Here's how the part is built. I have some questions about the finished solid (model axes, mm). Face numbers are marked on the shaded views. A direction names the side the tool comes from. Round coordinates to 2 decimals unless told otherwise and drop trailing zeros. Order: outer loops, then holes, each group sorted by start corner. A loop starts at its lowest first (then second) coordinate and runs counter-clockwise, first axis right, second up. Notation, with made-up numbers: M 37.25,54 L 64.25,54 A27 cw 64.25,90 Z; hole C 54.25,25 d9. An arc over 180 degrees is marked long. Write item = value, one per line. Start each with the question number.
Item 1: I'm going to push a flat-ended pin straight in: P1, Ø1, axis at y = 1.5, z = 0, coming from the -X side. Where does the tip first touch, or does it pass through?
Item 2: I want a section at C-C, the plane y = 1.95. State how many separate pieces and enclosed holes the cut face has, plus the area to 3 significant figures.
Item 3: We'd pull the mould along Z, two halves only. Please class the marked faces 4, 5 and 6: pulls with the +Z half, pulls with the -Z half, needs draft (parallel to the pull), parting line crosses it, or undercut.
Item 4: I want a section at B-B, the plane z = 0. List the corners of the cut face in (x, y) for me (1 decimal).
Item 5: For the marked faces 1, 2 and 3, which set-ups out of +Z, -Z, +X, -X, +Y, -Y let a thin tool reach every point of the face, with its end or its side?
Item 6: I want a section at D-D, the plane z = 12.5. List the corners of the cut face in (x, y) for me (3 decimals).
Item 7: I want a section at A-A, the plane x = 0. List the corners of the cut face in (y, z) for me (3 decimals).
Item 8: Please list where these lines run through material, in increasing order: L1, parallel to X at y = 0.9, z = 0; L2, parallel to Z at x = 0, y = 2.35; L3, parallel to X at y = 1.25, z = -0.5.
```python
from build123d import *

# Parameters (mm, degrees)
BOSS_EXTRUDE1_DEPTH = 3.175
SKETCH2_R           = 1.143
SKETCH2_R_2         = 2.54
CUT_EXTRUDE1_DEPTH  = 3.175


with BuildPart() as part:
    # Sketch1 → Boss-Extrude1 (new body)
    with BuildSketch(Plane(origin=(0, 0, 0), x_dir=(1, 0, 0), z_dir=(0, 1, 0))):
        with BuildLine():
            Line((0.635, 18.750209072), (-0.635, 18.750209114))
            Line((-0.635, 18.750209114), (-1.33510965, 16.137364669))
            ThreePointArc((-1.33510965, 16.137364669), (-1.951790294, 16.074438432), (-2.565610552, 15.987954802))
            Line((-2.565610552, 15.987954802), (-3.870670686, 18.357327521))
            Line((-3.870670686, 18.357327521), (-5.103766804, 18.053396667))
            Line((-5.103766804, 18.053396667), (-5.158237936, 15.348929528))
            ThreePointArc((-5.158237936, 15.348929528), (-5.741939727, 15.140250474), (-6.317226596, 14.909383099))
            Line((-6.317226596, 14.909383099), (-8.15139206, 16.897584819))
            Line((-8.15139206, 16.897584819), (-9.275921232, 16.307386428))
            Line((-9.275921232, 16.307386428), (-8.681588182, 13.668470393))
            ThreePointArc((-8.681588182, 13.668470393), (-9.198388493, 13.326166192), (-9.701708393, 12.964332243))
            Line((-9.701708393, 12.964332243), (-11.958384157, 14.455815909))
            Line((-11.958384157, 14.455815909), (-12.908992835, 13.613650164))
            Line((-12.908992835, 13.613650164), (-11.70039608, 11.193649442))
            ThreePointArc((-11.70039608, 11.193649442), (-12.120260356, 10.737613569), (-12.522362162, 10.265841521))
            Line((-12.522362162, 10.265841521), (-15.070398434, 11.173927523))
            Line((-15.070398434, 11.173927523), (-15.791840697, 10.128738036))
            Line((-15.791840697, 10.128738036), (-14.039219486, 8.068294272))
            ThreePointArc((-14.039219486, 8.068294272), (-14.337746742, 7.525029875), (-14.615261759, 6.970737405))
            Line((-14.615261759, 6.970737405), (-17.306575933, 7.242651084))
            Line((-17.306575933, 7.242651084), (-17.756924178, 6.055180471))
            Line((-17.756924178, 6.055180471), (-15.562134487, 4.474039167))
            ThreePointArc((-15.562134487, 4.474039167), (-15.721975403, 3.875118797), (-15.858775467, 3.270519368))
            Line((-15.858775467, 3.270519368), (-18.536958145, 2.890458091))
            Line((-18.536958145, 2.890458091), (-18.69003977, 1.629717826))
            Line((-18.69003977, 1.629717826), (-16.180634797, 0.619769168))
            ThreePointArc((-16.180634797, 0.619769168), (-16.1925, -1e-07), (-16.180634789, -0.619769367))
            Line((-16.180634789, -0.619769367), (-18.690039729, -1.629717821))
            Line((-18.690039729, -1.629717821), (-18.536958186, -2.890458096))
            Line((-18.536958186, -2.890458096), (-15.858775427, -3.270519563))
            ThreePointArc((-15.858775427, -3.270519563), (-15.721975355, -3.875118991), (-15.562134432, -4.474039358))
            Line((-15.562134432, -4.474039358), (-17.75692414, -6.055180456))
            Line((-17.75692414, -6.055180456), (-17.306575972, -7.242651099))
            Line((-17.306575972, -7.242651099), (-14.615261673, -6.970737585))
            ThreePointArc((-14.615261673, -6.970737585), (-14.337746649, -7.525030051), (-14.039219387, -8.068294445))
            Line((-14.039219387, -8.068294445), (-15.791840663, -10.128738013))
            Line((-15.791840663, -10.128738013), (-15.070398469, -11.173927546))
            Line((-15.070398469, -11.173927546), (-12.522362036, -10.265841675))
            ThreePointArc((-12.522362036, -10.265841675), (-12.120260224, -10.737613718), (-11.700395942, -11.193649586))
            Line((-11.700395942, -11.193649586), (-12.908992808, -13.613650133))
            Line((-12.908992808, -13.613650133), (-11.958384185, -14.45581594))
            Line((-11.958384185, -14.45581594), (-9.701708233, -12.964332363))
            ThreePointArc((-9.701708233, -12.964332363), (-9.198388329, -13.326166305), (-8.681588014, -13.6684705))
            Line((-8.681588014, -13.6684705), (-9.275921213, -16.307386391))
            Line((-9.275921213, -16.307386391), (-8.15139208, -16.897584856))
            Line((-8.15139208, -16.897584856), (-6.317226413, -14.909383176))
            ThreePointArc((-6.317226413, -14.909383176), (-5.74193954, -15.140250545), (-5.158237747, -15.348929591))
            Line((-5.158237747, -15.348929591), (-5.103766794, -18.053396627))
            Line((-5.103766794, -18.053396627), (-3.870670696, -18.357327561))
            Line((-3.870670696, -18.357327561), (-2.565610355, -15.987954833))
            ThreePointArc((-2.565610355, -15.987954833), (-1.951790096, -16.074438456), (-1.335109452, -16.137364686))
            Line((-1.335109452, -16.137364686), (-0.635, -18.750209072))
            Line((-0.635, -18.750209072), (0.635, -18.750209114))
            Line((0.635, -18.750209114), (1.33510965, -16.137364669))
            ThreePointArc((1.33510965, -16.137364669), (1.951790294, -16.074438432), (2.565610552, -15.987954802))
            Line((2.565610552, -15.987954802), (3.870670686, -18.357327521))
            Line((3.870670686, -18.357327521), (5.103766804, -18.053396667))
            Line((5.103766804, -18.053396667), (5.158237936, -15.348929528))
            ThreePointArc((5.158237936, -15.348929528), (5.741939727, -15.140250474), (6.317226596, -14.909383099))
            Line((6.317226596, -14.909383099), (8.15139206, -16.897584819))
            Line((8.15139206, -16.897584819), (9.275921232, -16.307386428))
            Line((9.275921232, -16.307386428), (8.681588182, -13.668470393))
            ThreePointArc((8.681588182, -13.668470393), (9.198388493, -13.326166192), (9.701708393, -12.964332243))
            Line((9.701708393, -12.964332243), (11.958384157, -14.455815909))
            Line((11.958384157, -14.455815909), (12.908992835, -13.613650164))
            Line((12.908992835, -13.613650164), (11.70039608, -11.193649442))
            ThreePointArc((11.70039608, -11.193649442), (12.120260356, -10.737613569), (12.522362162, -10.265841521))
            Line((12.522362162, -10.265841521), (15.070398434, -11.173927523))
            Line((15.070398434, -11.173927523), (15.791840697, -10.128738036))
            Line((15.791840697, -10.128738036), (14.039219486, -8.068294272))
            ThreePointArc((14.039219486, -8.068294272), (14.337746742, -7.525029875), (14.615261759, -6.970737405))
            Line((14.615261759, -6.970737405), (17.306575933, -7.242651084))
            Line((17.306575933, -7.242651084), (17.756924178, -6.055180471))
            Line((17.756924178, -6.055180471), (15.562134487, -4.474039167))
            ThreePointArc((15.562134487, -4.474039167), (15.721975403, -3.875118797), (15.858775467, -3.270519368))
            Line((15.858775467, -3.270519368), (18.536958145, -2.890458091))
            Line((18.536958145, -2.890458091), (18.69003977, -1.629717826))
            Line((18.69003977, -1.629717826), (16.180634797, -0.619769168))
            ThreePointArc((16.180634797, -0.619769168), (16.1925, 1e-07), (16.180634789, 0.619769367))
            Line((16.180634789, 0.619769367), (18.690039729, 1.629717821))
            Line((18.690039729, 1.629717821), (18.536958186, 2.890458096))
            Line((18.536958186, 2.890458096), (15.858775427, 3.270519563))
            ThreePointArc((15.858775427, 3.270519563), (15.721975355, 3.875118991), (15.562134432, 4.474039358))
            Line((15.562134432, 4.474039358), (17.75692414, 6.055180456))
            Line((17.75692414, 6.055180456), (17.306575972, 7.242651099))
            Line((17.306575972, 7.242651099), (14.615261673, 6.970737585))
            ThreePointArc((14.615261673, 6.970737585), (14.337746649, 7.525030051), (14.039219387, 8.068294445))
            Line((14.039219387, 8.068294445), (15.791840663, 10.128738013))
            Line((15.791840663, 10.128738013), (15.070398469, 11.173927546))
            Line((15.070398469, 11.173927546), (12.522362036, 10.265841675))
            ThreePointArc((12.522362036, 10.265841675), (12.120260224, 10.737613718), (11.700395942, 11.193649586))
            Line((11.700395942, 11.193649586), (12.908992808, 13.613650133))
            Line((12.908992808, 13.613650133), (11.958384185, 14.45581594))
            Line((11.958384185, 14.45581594), (9.701708233, 12.964332363))
            ThreePointArc((9.701708233, 12.964332363), (9.198388329, 13.326166305), (8.681588014, 13.6684705))
            Line((8.681588014, 13.6684705), (9.275921213, 16.307386391))
            Line((9.275921213, 16.307386391), (8.15139208, 16.897584856))
            Line((8.15139208, 16.897584856), (6.317226413, 14.909383176))
            ThreePointArc((6.317226413, 14.909383176), (5.74193954, 15.140250545), (5.158237747, 15.348929591))
            Line((5.158237747, 15.348929591), (5.103766794, 18.053396627))
            Line((5.103766794, 18.053396627), (3.870670696, 18.357327561))
            Line((3.870670696, 18.357327561), (2.565610355, 15.987954833))
            ThreePointArc((2.565610355, 15.987954833), (1.951790096, 16.074438456), (1.335109452, 16.137364686))
            Line((1.335109452, 16.137364686), (0.635, 18.750209072))
        make_face()
    extrude(amount=BOSS_EXTRUDE1_DEPTH)

    # Sketch2 → Cut-Extrude1 (cut)
    with BuildSketch(Plane(origin=(0, 0, 0), x_dir=(1, 0, 0), z_dir=(0, 1, 0))):
        with Locations((-5.08, 0)):
            Circle(SKETCH2_R)
        with Locations((0, 5.08)):
            Circle(SKETCH2_R)
        with Locations((5.08, 0)):
            Circle(SKETCH2_R)
        with Locations((0, -5.08)):
            Circle(SKETCH2_R)
        Circle(SKETCH2_R_2)
    extrude(amount=CUT_EXTRUDE1_DEPTH, mode=Mode.SUBTRACT)


solid = part.part
```
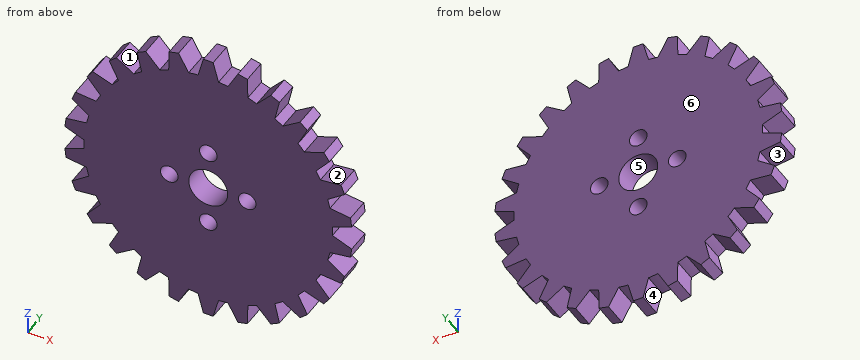
Filled in:
q1.P1 = -16.19
q2.separate_pieces = 1
q2.enclosed_holes = 5
q2.area = 918 mm^2
q3.face_4 = pulls with the -Z half
q3.face_5 = undercut
q3.face_6 = needs draft
q4.outline = M -16.2,0 L -6.2,0 L -6.2,3.2 L -16.2,3.2 Z; M -3.9,0 L -2.5,0 L -2.5,3.2 L -3.9,3.2 Z; M 2.5,0 L 3.9,0 L 3.9,3.2 L 2.5,3.2 Z; M 6.2,0 L 16.2,0 L 16.2,3.2 L 6.2,3.2 Z
q5.face_1 = +Z, +Y, -Y
q5.face_2 = +Y, -Y
q5.face_3 = -X, +Y, -Y
q6.outline = M -12.353,0 L 12.353,0 L 12.353,3.175 L -12.353,3.175 Z
q7.outline = M 0,-18.75 L 3.175,-18.75 L 3.175,-6.223 L 0,-6.223 Z; M 0,-3.937 L 3.175,-3.937 L 3.175,-2.54 L 0,-2.54 Z; M 0,2.54 L 3.175,2.54 L 3.175,3.937 L 0,3.937 Z; M 0,6.223 L 3.175,6.223 L 3.175,18.75 L 0,18.75 Z
q8.L1 = -16.19 to -6.22, -3.94 to -2.54, 2.54 to 3.94, 6.22 to 16.19
q8.L2 = -18.75 to -6.22, -3.94 to -2.54, 2.54 to 3.94, 6.22 to 18.75
q8.L3 = -16.18 to -6.11, -4.05 to -2.49, 2.49 to 4.05, 6.11 to 16.18
